from build123d import *

# Parameters (mm, degrees)
SKETCH1_W           = 47.498
SKETCH1_H           = 38.1
BOSS_EXTRUDE1_DEPTH = 63.5
SKETCH3_W           = 47.498
SKETCH3_H           = 10.16
CUT_EXTRUDE1_DEPTH  = 38.1
SKETCH4_W           = 41.91
SKETCH4_H           = 17.145
CUT_EXTRUDE2_DEPTH  = 19.05
SKETCH5_W           = 40.132
SKETCH5_H           = 10.16
CUT_EXTRUDE3_DEPTH  = 49.770149692
SKETCH6_W           = 2.286
SKETCH6_H           = 38.1
CUT_EXTRUDE4_DEPTH  = 31.75


with BuildPart() as part:
    # Sketch1 → Boss-Extrude1 (new body)
    with BuildSketch(Plane(origin=(0, 0, 0), x_dir=(1, 0, 0), z_dir=(0, 1, 0))):
        Rectangle(SKETCH1_W, SKETCH1_H)
    extrude(amount=BOSS_EXTRUDE1_DEPTH)

    # Sketch3 → Cut-Extrude1 (cut)
    with BuildSketch(Plane(origin=(0, 63.5, 0), x_dir=(1, 0, 0), z_dir=(0, 1, 0))):
        Rectangle(SKETCH3_W, SKETCH3_H)
    extrude(amount=-CUT_EXTRUDE1_DEPTH, mode=Mode.SUBTRACT)

    # Sketch4 → Cut-Extrude2 (cut)
    with BuildSketch(Plane.XZ):
        with Locations((-2.794, 0)):
            Rectangle(SKETCH4_W, SKETCH4_H)
    extrude(amount=-CUT_EXTRUDE2_DEPTH, mode=Mode.SUBTRACT)

    # Sketch5 → Cut-Extrude3 (cut, through all)
    with BuildSketch(Plane(origin=(0, 25.4, 0), x_dir=(1, 0, 0), z_dir=(0, 1, 0))):
        with Locations((-1.905, 0)):
            Rectangle(SKETCH5_W, SKETCH5_H)
    extrude(amount=-CUT_EXTRUDE3_DEPTH, mode=Mode.SUBTRACT)

    # Sketch6 → Cut-Extrude4 (cut)
    with BuildSketch(Plane(origin=(0, 63.5, 0), x_dir=(1, 0, 0), z_dir=(0, 1, 0))):
        with Locations((-22.606, 0)):
            Rectangle(SKETCH6_W, SKETCH6_H)
    extrude(amount=-CUT_EXTRUDE4_DEPTH, mode=Mode.SUBTRACT)


solid = part.part
Design review of the part built by this model. Coordinates are the model's own, in mm. A direction names the side the tool comes from. Give positions to 0.01 mm unless a question says otherwise; leave off trailing zeros. Order: outer loops, then holes, each group sorted by start corner. A loop starts at its lowest first (then second) coordinate and runs counter-clockwise, first axis right, second up.
1. Add section C-C, the plane x = 4.5. State the section outline as (y, z) points, then the cut area to 3 significant figures.
Solution:
outline: (0, -19.05) - (63.5, -19.05) - (63.5, -5.08) - (19.05, -5.08) - (19.05, -8.57) - (0, -8.57) - close; (0, 8.57) - (19.05, 8.57) - (19.05, 5.08) - (63.5, 5.08) - (63.5, 19.05) - (0, 19.05) - close
area: 1,640 mm2
2. Add section B-B, the plane z = 4. State the section outline as (x, y) points.
Solution:
outline: (-23.75, 19.05) - (-21.97, 19.05) - (-21.97, 25.4) - (-23.75, 25.4) - close; (18.16, 0) - (23.75, 0) - (23.75, 25.4) - (18.16, 25.4) - close
3. For pin 1 Ø10 at (x, z) = (13, -3.5) entering from -Y; pin 2 Ø3 at (x, z) = (21.5, -2) entering from +Y; pin 3 Ø13.5 at (y, z) = (11.5, 3) entering from -X; pin 4 Ø4 at (y, z) = (48, -10.5) entering from -X, all flat-tipped, find the tip position at first contact; note any pin that passes through.
Solution:
pin 1: stops at y = 19.05
pin 2: stops at y = 25.4
pin 3: stops at x = -23.75
pin 4: stops at x = -21.46
4. Add section D-D, the plane y = 7. State the section outline as (x, z) points.
Solution:
outline: (-23.75, -19.05) - (23.75, -19.05) - (23.75, 19.05) - (-23.75, 19.05) - (-23.75, 8.57) - (18.16, 8.57) - (18.16, -8.57) - (-23.75, -8.57) - close
5. To check wall thickness, follow L1, parallel to Z at x = 13, y = 27; L2, parallel to Z at x = 2, y = 9; L3, parallel to X at y = 34, z = -8.5. State the ranges of each line that lie inside material, in increasing order.
Solution:
L1: z = -19.05 to -5.08, 5.08 to 19.05
L2: z = -19.05 to -8.57, 8.57 to 19.05
L3: x = -21.46 to 23.75
6. Mouldability with a two-part tool opening along X and no side actions: class faces 4 (the flat face through (-21.971, 22, 0)), 5 (the flat face through (0, 31, -19.05)), 6 (the flat face through (-23.749, 23, 0)) as +X half, -X half, draft (parallel to the pull), parting line (faces both ways), or undercut.
Solution:
face 4: undercut
face 5: draft
face 6: -X half
7. Add section A-A, the plane y = 29. State the section outline as (x, z) points, then the cut area to 3 significant figures.
Solution:
outline: (-23.75, -19.05) - (23.75, -19.05) - (23.75, -5.08) - (-23.75, -5.08) - close; (-23.75, 5.08) - (23.75, 5.08) - (23.75, 19.05) - (-23.75, 19.05) - close
area: 1,330 mm2
8. Tool access review of faces 1 (the flat face through (-3, 19.05, 6)), 2 (the flat face through (-23, 31.75, -12)), 3 (the flat face through (21, 25.4, 0)): name each direction out of +Z, -Z, +X, -X, +Y, -Y from which nothing blocks a thin tool from reaching the whole face with its end or side.
Solution:
face 1: -X, -Y
face 2: +Z, -Z, -X, +Y
face 3: +X, -X, +Y
